```python
from build123d import *

# Parameters (mm, degrees)
SKETCH3_W           = 50.8
SKETCH3_H           = 25.4
SKETCH3_R           = 2.00025
SKETCH3_R_2         = 5.715
BOSS_EXTRUDE1_DEPTH = 1.5875
SKETCH4_W           = 50.8
SKETCH4_H           = 2.54
BOSS_EXTRUDE2_DEPTH = 11.43


with BuildPart() as part:
    # Sketch3 → Boss-Extrude1 (new, symmetric)
    with BuildSketch(Plane(origin=(0, 0, 0), x_dir=(0, 0, -1), z_dir=(1, 0, 0))):
        Rectangle(SKETCH3_W, SKETCH3_H)
        with Locations((-17.5006, 4.191)):
            Circle(SKETCH3_R, mode=Mode.SUBTRACT)
        with Locations((17.5006, 4.191)):
            Circle(SKETCH3_R, mode=Mode.SUBTRACT)
        with Locations((0, -3.81)):
            Circle(SKETCH3_R_2, mode=Mode.SUBTRACT)
    extrude(amount=BOSS_EXTRUDE1_DEPTH, both=True)

    # Sketch4 → Boss-Extrude2 (add, symmetric)
    with BuildSketch(Plane(origin=(0, 0, 0), x_dir=(0, 0, -1), z_dir=(1, 0, 0))):
        with Locations((0, -11.43)):
            Rectangle(SKETCH4_W, SKETCH4_H)
    extrude(amount=BOSS_EXTRUDE2_DEPTH, both=True)


solid = part.part
```
For this review, take the finished solid that the model builds, in its own axes (mm). A direction names the side the tool comes from. Round coordinates to 2 decimals unless told otherwise and drop trailing zeros. Write each loop counter-clockwise with the first axis right and the second up, starting at its lowest first coordinate (ties: lowest second). Pieces come first, ordered by that corner, then holes. Notation, with made-up numbers: (68.25, 0.5) -> (116.25, 0.5) arc R27 cw to (116.25, 32.5) -> close; hole circle Ø11 at (51, 17.5). An arc over 180 degrees is marked (long way). Use one line per item in the form item = value.
1) Tool access review of faces 4 (the flat face through (11.43, -11, 0)), 5 (the flat face through (-6, -10.16, 0)), 6 (the flat face through (1.588, 4, 0)): name each direction out of +Z, -Z, +X, -X, +Y, -Y from which nothing blocks a thin tool from reaching the whole face with its end or side.
Found:
face_4 = +Z, -Z, +X, +Y, -Y
face_5 = +Z, -Z, -X, +Y
face_6 = +Z, -Z, +X, +Y
2) Mouldability with a two-part tool opening along Y and no side actions: class faces 1 (the flat face through (0, -12.7, 0)), 2 (the flat face through (0, 12.7, 0)), 3 (the cylindrical face through (-0.022, 2.238, -17.067)) as +Y half, -Y half, draft (parallel to the pull), parting line (faces both ways), or undercut.
Found:
face_1 = -Y half
face_2 = +Y half
face_3 = undercut
3) Take a section at B-B, the plane y = -3.81. Write out the cut boundary in (x, z) (1 decimal).
Found:
outline = (-1.6, -25.4) -> (1.6, -25.4) -> (1.6, -5.7) -> (-1.6, -5.7) -> close; (-1.6, 5.7) -> (1.6, 5.7) -> (1.6, 25.4) -> (-1.6, 25.4) -> close
4) Take a section at C-C, the plane y = 5. Write out the cut boundary in (x, z), and give its area (3 significant figures).
Found:
outline = (-1.59, -25.4) -> (1.59, -25.4) -> (1.59, -19.33) -> (-1.59, -19.33) -> close; (-1.59, -15.67) -> (1.59, -15.67) -> (1.59, 15.67) -> (-1.59, 15.67) -> close; (-1.59, 19.33) -> (1.59, 19.33) -> (1.59, 25.4) -> (-1.59, 25.4) -> close
area = 138 mm2
5) Clearance check with flat-ended pins moving along their axes: pin 1 (11.5 mm diameter, centred on y = 4, z = -7.5, fed in from -X); pin 2 (11.5 mm diameter, centred on y = -0.5, z = -6.5, fed in from +X); pin 3 (5 mm diameter, centred on x = 5, z = 8, fed in from +Y). State where each tip first meets the part, or that it passes through.
Found:
pin_1 = -1.59
pin_2 = 1.59
pin_3 = -10.16
6) Take a section at A-A, the plane z = 0. Write out the cut boundary in (x, y) (1 decimal).
Found:
outline = (-11.4, -12.7) -> (11.4, -12.7) -> (11.4, -10.2) -> (1.6, -10.2) -> (1.6, -9.5) -> (-1.6, -9.5) -> (-1.6, -10.2) -> (-11.4, -10.2) -> close; (-1.6, 1.9) -> (1.6, 1.9) -> (1.6, 12.7) -> (-1.6, 12.7) -> close
7) Take a section at D-D, the plane z = -12.5. Write out the cut boundary in (x, y), and give its area (3 significant figures).
Found:
outline = (-11.43, -12.7) -> (11.43, -12.7) -> (11.43, -10.16) -> (1.59, -10.16) -> (1.59, 12.7) -> (-1.59, 12.7) -> (-1.59, -10.16) -> (-11.43, -10.16) -> close
area = 131 mm2
8) To check wall thickness, follow L1, parallel to Y at x = -0.15, z = 0 (3 decimals); L2, parallel to X at y = 3, z = -5; L3, parallel to Y at x = 2, z = -4. State the ranges of each line that lie inside material, in increasing order. Write a range as from..to.
Found:
L1 = -12.7..-9.525, 1.905..12.7
L2 = -1.59..1.59
L3 = -12.7..-10.16
